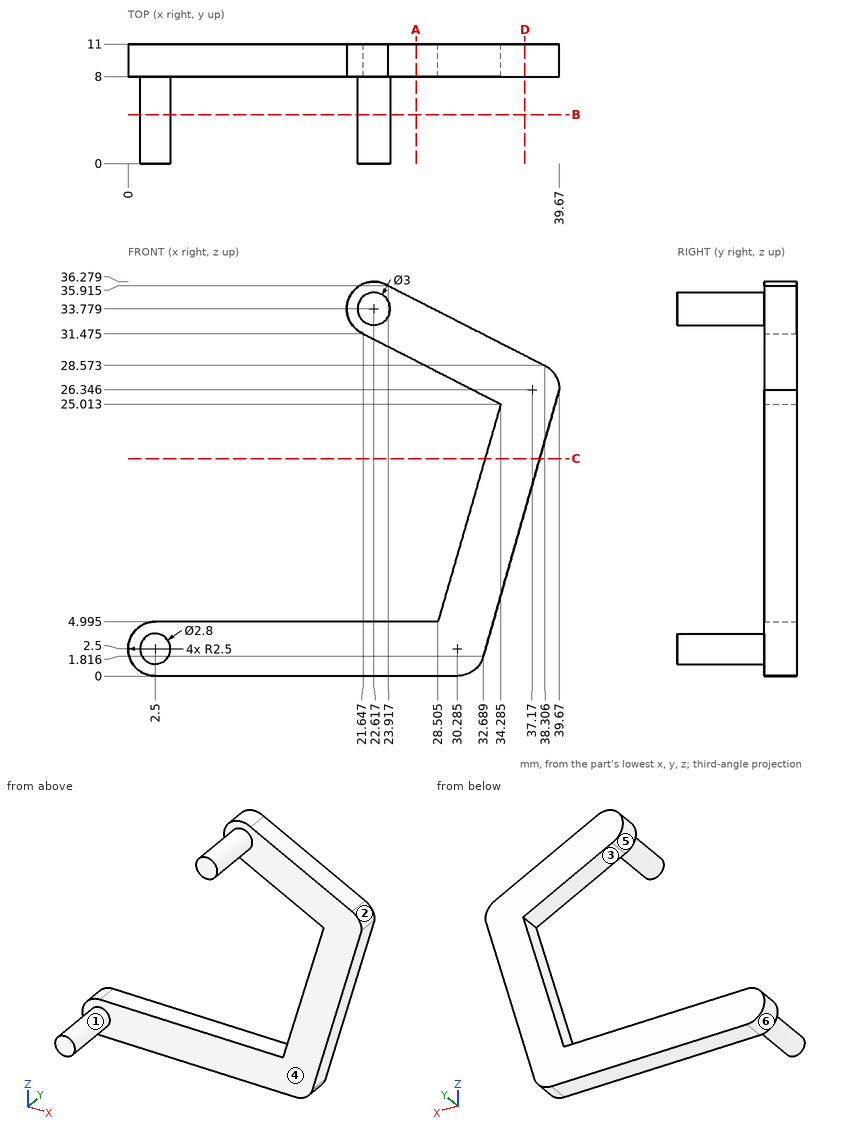
Can you work these out from the drawing? Everything is in mm from the part's minimum corner. A direction names the side the tool comes from. Round coordinates to 2 decimals unless told otherwise and drop trailing zeros. Write each loop counter-clockwise with the first axis right and the second up, starting at its lowest first coordinate (ties: lowest second). Pieces come first, ordered by that corner, then holes. Notation, with made-up numbers: (85, 65) - (103, 65) arc R26 cw to (103, 85) - close; hole circle Ø4 at (23, 87.25). An arc over 180 degrees is marked (long way). Write each question's results on one line, items separated by ' | '. Start each with the question number.
1) Suppose I cut it at D-D (x = 36.5). List the corners of the cut face in (y, z) for me (1 decimal).
2) Please list where these lines run through material, in increasing order: line 1 (Z direction, x = 14.5, y = 8.25); line 2 (Z direction, x = 23.5, y = 2) (1 decimal); line 3 (Z direction, x = 22, y = 9.25) (1 decimal).
3) Suppose I cut it at A-A (x = 26.5). List the corners of the cut face in (y, z) for me (1 decimal).
4) For pin 1 Ø5 at (x, y) = (25.5, 4.5) entering from -Z; pin 2 Ø1.5 at (y, z) = (5, 32) entering from -X (1 decimal); pin 3 Ø3 at (y, z) = (9.5, 24) entering from -X (1 decimal), each with a flat end and sliding along its axis, tell me the tip position at first contact or that it passes through.
5) Which directions (+Z, -Z, +X, -X, +Y, -Y) give clear straight access to the entire face, cutting with the end or side of a thin tool? Please do the marked faces 1, 2 and 3.
6) Suppose I cut it at C-C (z = 20). List the corners of the cut face in (x, y) for me.
7) We'd pull the mould along Z, two halves only. Please class the marked faces 4, 5 and 6: released by +Z, released by -Z, zero draft, split by the parting line, or undercut.
8) Suppose I cut it at B-B (y = 4.5). List the corners of the cut face in (x, z) for me.
Here are the results:
1) outline: (8, 15.2) - (11, 15.2) - (11, 29.5) - (8, 29.5) - close
2) line 1: z = 0 to 5 | line 2: z = 32.6 to 35 | line 3: z = 0 to 5, 31.3 to 36.2
3) outline: (8, 0) - (11, 0) - (11, 5) - (8, 5) - close; (8, 29) - (11, 29) - (11, 34.6) - (8, 34.6) - close
4) pin 1: stops at z = 32.33 | pin 2: stops at x = 21.5 | pin 3: stops at x = 33.3
5) face 1: -Y | face 2: +Z, +X, +Y, -Y | face 3: -X, +Y, -Y
6) outline: (32.84, 8) - (37.86, 8) - (37.86, 11) - (32.84, 11) - close
7) face 4: zero draft | face 5: undercut | face 6: split by the parting line
8) outline: circle Ø2.8 at (2.5, 2.5); circle Ø3 at (22.62, 33.78)
